```python
from build123d import *

# Parameters (mm, degrees)
F1_DEPTH  = 25
F5_D      = 4.2
F5_DEPTH  = 20
F5_TIP    = 1.2618073
F10_DEPTH = 50.001


with BuildPart() as f1:
    # F0 (on Front) → F1 (new body, symmetric)
    with BuildSketch(Plane.XZ):
        with BuildLine():
            ThreePointArc((0, 315), (37.7725508345, 312.7270925319), (75, 305.9411708156))
            Line((75, 305.9411708156), (75, 335))
            Line((75, 335), (0, 335))
            Line((0, 335), (0, 315))
        make_face()
        with BuildLine():
            ThreePointArc((-75, 305.9411708156), (-37.7725508345, 312.7270925319), (0, 315))
            Line((0, 315), (0, 335))
            Line((0, 335), (-75, 335))
            Line((-75, 335), (-75, 305.9411708156))
        make_face()
    extrude(amount=F1_DEPTH, both=True)

    # F2 (on face) → F3 (revolve, cut)
    with BuildSketch(Plane.XY.offset(335)):
        with BuildLine():
            Line((-13.2664991614, 7), (-75, 7))
            Line((-75, 7), (-75, 0))
            Line((-75, 0), (-15, 0))
            ThreePointArc((-15, 0), (-14.5601766373, 3.6057254872), (-13.2664991614, 7))
        make_face()
        with BuildLine():
            ThreePointArc((13.2664991614, 7), (0, 15), (-13.2664991614, 7))
            ThreePointArc((-13.2664991614, 7), (-14.5601766373, 3.6057254872), (-15, 0))
            Line((-15, 0), (-13.2664991614, 0))
            Line((-13.2664991614, 0), (13.2664991614, 0))
            Line((13.2664991614, 0), (15, 0))
            ThreePointArc((15, 0), (14.5601766373, 3.6057254872), (13.2664991614, 7))
        make_face()
        with BuildLine():
            Line((75, 7), (13.2664991614, 7))
            ThreePointArc((13.2664991614, 7), (14.5601766373, 3.6057254872), (15, 0))
            Line((15, 0), (75, 0))
            Line((75, 0), (75, 7))
        make_face()
    revolve(axis=Axis((-44.1332495807, 0, 335), (1, 0, 0)), mode=Mode.SUBTRACT)

    # F5
    with Locations(Plane.XY.offset(335)):
        with Locations((-70, 20), (-70, -20), (70, 20), (70, -20)):
            Hole(F5_D / 2, depth=F5_DEPTH)
            with Locations((0, 0, -(F5_DEPTH + F5_TIP / 2))):  # 118° drill point
                Cone(0, F5_D / 2, F5_TIP, mode=Mode.SUBTRACT)

    # F6 (on face) → F7 (revolve, cut)
    with BuildSketch(Plane.XY.offset(335)):
        with BuildLine():
            Line((0, 0), (-5, 0))
            Line((-5, 0), (-5, -14.1421356237))
            ThreePointArc((-5, -14.1421356237), (-2.5365296809, -14.7839783948), (0, -15))
            Line((0, -15), (0, 0))
        make_face()
        with BuildLine():
            ThreePointArc((0, -15), (-2.5365296809, -14.7839783948), (-5, -14.1421356237))
            Line((-5, -14.1421356237), (-5, -25))
            Line((-5, -25), (0, -25))
            Line((0, -25), (0, -15))
        make_face()
    revolve(axis=Axis((0, -12.5, 335), (0, -1, 0)), mode=Mode.SUBTRACT)

    # F9 (on face) → F10 (cut, through all)
    with BuildSketch(Plane.XZ.offset(25)):
        with BuildLine():
            ThreePointArc((0, 315), (37.7725508345, 312.7270925319), (75, 305.9411708156))
            Line((75, 305.9411708156), (75, 315))
            Line((75, 315), (0, 315))
        make_face()
        with BuildLine():
            Line((-75, 315), (-75, 305.9411708156))
            ThreePointArc((-75, 305.9411708156), (-37.7725508345, 312.7270925319), (0, 315))
            Line((0, 315), (-75, 315))
        make_face()
    extrude(amount=-F10_DEPTH, mode=Mode.SUBTRACT)


solid = f1.part
```
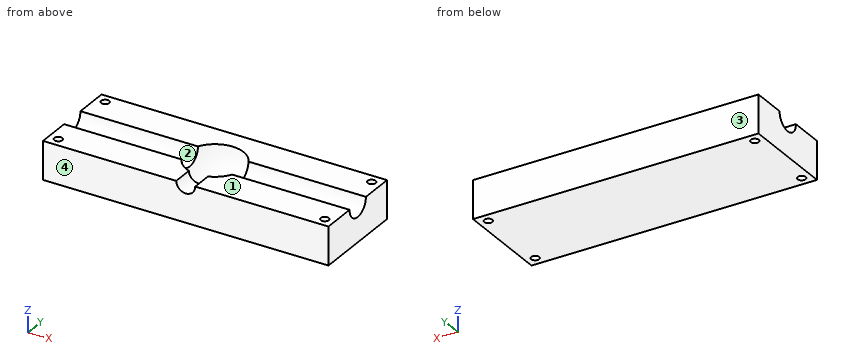
Could you check a few things on this model? Use its own coordinates, in mm. Face numbers are marked on the shaded views. Give positions to 0.01 mm unless a question says otherwise; leave off trailing zeros. Write each loop counter-clockwise with the first axis right and the second up, starting at its lowest first coordinate (ties: lowest second). Pieces come first, ordered by that corner, then holes. Notation, with made-up numbers: (-24.75, 17.5) - (9.25, 17.5) arc R28 ccw to (9.25, 53.5) - close; hole circle Ø1 at (48.5, 80.5). An arc over 180 degrees is marked (long way). One line per item, written item: value. Start each with the question number.
Item 1: If we mould it in two halves opening along Y, with no side actions, what happens to the marked faces 1, 2, 3 and 4? For each: +Y half, -Y half, draft (parallel to the pull), parting line (faces both ways), or undercut.
Item 2: I'm going to push a flat-ended pin straight in: pin 1 (4 mm diameter, centred on x = -70, y = 20, fed in from +Z). Where does the tip first touch, or does it pass through?
Item 3: Imagine slicing it at C-C, the plane y = 20. List the corners of the cut face in (x, z) for me.
Item 4: Please list where these lines run through material, in increasing order: line 1 (X direction, y = -20, z = 329.25); line 2 (Y direction, x = 70, z = 321.75); line 3 (Y direction, x = -17, z = 332). Write a range as from..to.
Item 5: Imagine slicing it at D-D, the plane x = -18.5. List the corners of the cut face in (y, z) for me.
Item 6: Imagine slicing it at A-A, the plane x = -70. List the corners of the cut face in (y, z) for me, and give its area (3 significant figures).
Item 7: Imagine slicing it at B-B, the plane y = -20. List the corners of the cut face in (x, z) for me.
Geometry says:
1. face 1: draft
1. face 2: undercut
1. face 3: +Y half
1. face 4: -Y half
2. pin 1: through
3. outline: (-75, 315) - (-72.1, 315) - (-72.1, 335) - (-75, 335) - close; (-67.9, 315) - (67.9, 315) - (67.9, 335) - (-67.9, 335) - close; (72.1, 315) - (75, 315) - (75, 335) - (72.1, 335) - close
4. line 1: -75..-72.1, -67.9..67.9, 72.1..75
4. line 2: -25..-22.1, -17.9..17.9, 22.1..25
4. line 3: -25..-6.32, 6.32..25
5. outline: (-25, 315) - (25, 315) - (25, 335) - (7, 335) arc R7 cw to (-7, 335) - (-25, 335) - close
6. outline: (-25, 315) - (-22.1, 315) - (-22.1, 335) - (-25, 335) - close; (-17.9, 315) - (17.9, 315) - (17.9, 335) - (7, 335) arc R7 cw to (-7, 335) - (-17.9, 335) - close; (22.1, 315) - (25, 315) - (25, 335) - (22.1, 335) - close
6. area: 755 mm^2
7. outline: (-75, 315) - (-72.1, 315) - (-72.1, 335) - (-75, 335) - close; (-67.9, 315) - (67.9, 315) - (67.9, 335) - (5, 335) arc R5 cw to (-5, 335) - (-67.9, 335) - close; (72.1, 315) - (75, 315) - (75, 335) - (72.1, 335) - close
